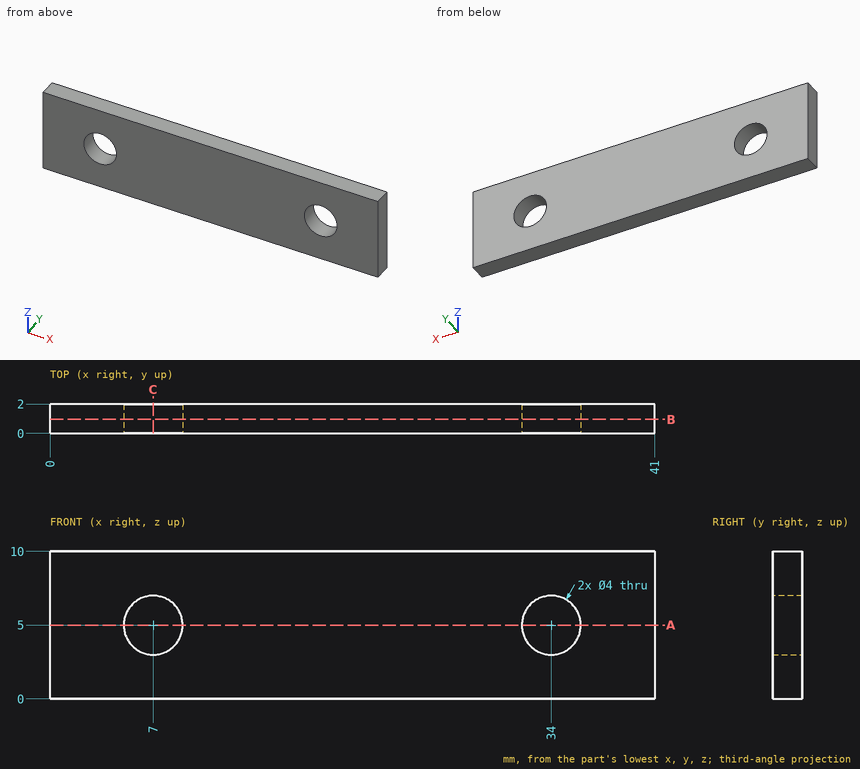
Geometry check sheet. Reference: drawing and pictorial views, mm from the part's lowest x, y, z. Round coordinates to 2 decimals unless told otherwise and drop trailing zeros. Loops run counter-clockwise (first coordinate to the right, second up) from the corner with the lowest first, then second, coordinate; pieces in that order, holes last. Notation, with made-up numbers: (-38, 24.5) - (-12, 24.5) arc R20 cw to (-12, 38.5) - close; hole circle Ø5 at (71.5, 85). An arc over 180 degrees is marked (long way). One line per question, with ' | ' between items. Start each with the question number.
1. Cross-section at B-B on y = 0.95. Record the cut outline in (x, z), then the cut area to 3 significant figures.
2. Cross-section at A-A on z = 5. Record the cut outline in (x, y).
3. Cross-section at C-C on x = 7. Record the cut outline in (y, z).
4. Scan lines: line 1 (X direction, y = 0.9, z = 5); line 2 (X direction, y = 1.4, z = 3.75); line 3 (Z direction, x = 8, y = 1.2). Record each from-to range of solid material in increasing order. Write a range as [from, to].
Taken from the geometry:
1) outline: (0, 0) - (41, 0) - (41, 10) - (0, 10) - close; hole circle Ø4 at (7, 5); hole circle Ø4 at (34, 5) | area: 385 mm²
2) outline: (0, 0) - (5, 0) - (5, 2) - (0, 2) - close; (9, 0) - (32, 0) - (32, 2) - (9, 2) - close; (36, 0) - (41, 0) - (41, 2) - (36, 2) - close
3) outline: (0, 0) - (2, 0) - (2, 3) - (0, 3) - close; (0, 7) - (2, 7) - (2, 10) - (0, 10) - close
4) line 1: [0, 5], [9, 32], [36, 41] | line 2: [0, 5.44], [8.56, 32.44], [35.56, 41] | line 3: [0, 3.27], [6.73, 10]
